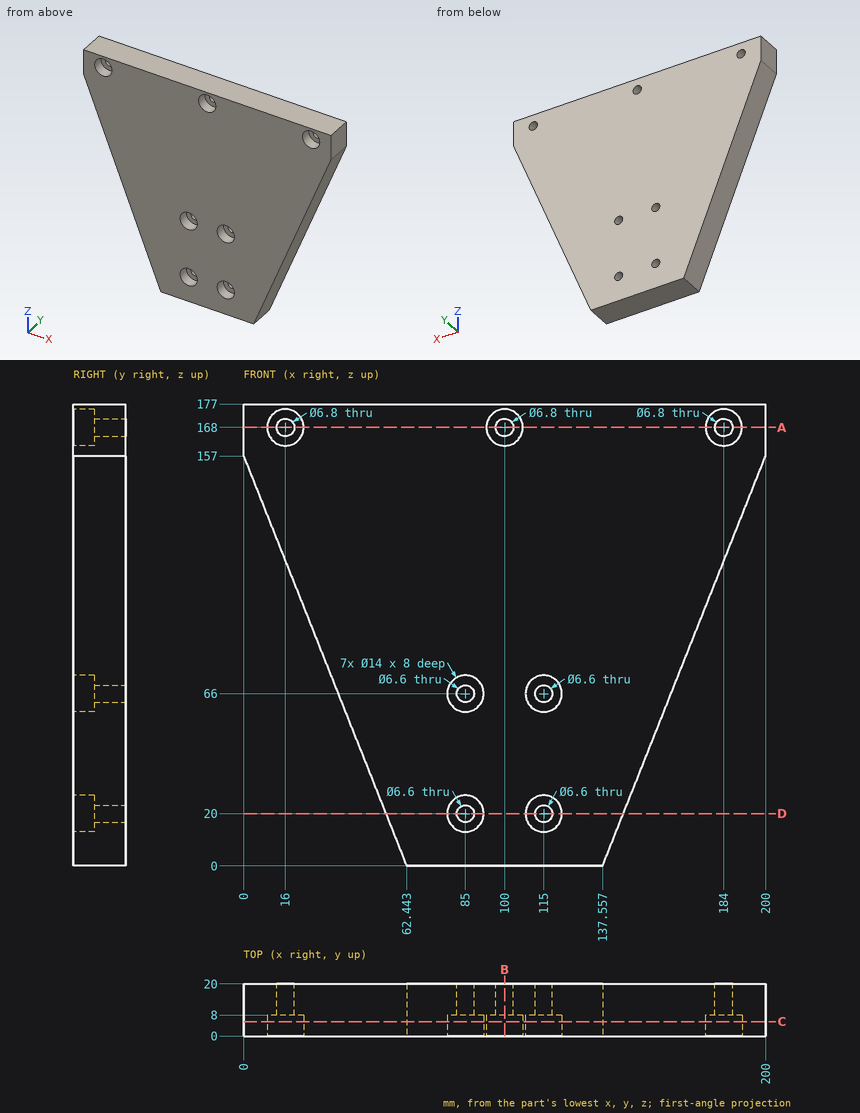
The drawing under review shows one solid part. Ordinate dimensions are in mm from its lowest x, y, z. Round coordinates to 2 decimals unless told otherwise and drop trailing zeros. Loops run counter-clockwise (first coordinate to the right, second up) from the corner with the lowest first, then second, coordinate; pieces in that order, holes last. Notation, with made-up numbers: (-7, 10.5) - (24, 10.5) arc R28 cw to (24, 32.5) - close; hole circle Ø10 at (24, 1). An arc over 180 degrees is marked (long way). Use a Markdown table: item, result. Add a question column.
Q1. Add section B-B (x = 100). State the section outline as (y, z) points, plus the area to 3 significant figures.
Q2. Add section A-A (z = 168). State the section outline as (x, y) points, plus the area to 3 significant figures.
Q3. Add section C-C (y = 5.5). State the section outline as (x, z) points, plus the area to 3 significant figures.
Q4. Insertion check: pin 1 Ø9 at (x, z) = (184, 168) entering from -Y; pin 2 Ø2 at (y, z) = (5, 107.5) entering from -X; pin 3 Ø1.5 at (y, z) = (7.5, 57.5) entering from +X (1 decimal); pin 4 Ø5.5 at (x, z) = (85, 66) entering from +Y. Each pin has a flat end and moves straight along its axis. Give the tip position at first contact, or say it passes through.
Q5. For probe 1 along X at (y, z) = (16.25, 168); probe 2 along X at (y, z) = (5.5, 24.5); probe 3 along Z at (x, y) = (97, 2) (1 decimal), list the stretches that pass through material, from the lowest coordinate up.
Q6. Add section D-D (z = 20). State the section outline as (x, y) points.
Worked answers:
| question | item | result |
|---|---|---|
| 1 | outline | (0, 0) - (20, 0) - (20, 164.6) - (8, 164.6) - (8, 161) - (0, 161) - close; (0, 175) - (8, 175) - (8, 171.4) - (20, 171.4) - (20, 177) - (0, 177) - close |
| 1 | area | 3,350 mm² |
| 2 | outline | (0, 0) - (9, 0) - (9, 8) - (12.6, 8) - (12.6, 20) - (0, 20) - close; (19.4, 8) - (23, 8) - (23, 0) - (93, 0) - (93, 8) - (96.6, 8) - (96.6, 20) - (19.4, 20) - close; (103.4, 8) - (107, 8) - (107, 0) - (177, 0) - (177, 8) - (180.6, 8) - (180.6, 20) - (103.4, 20) - close; (187.4, 8) - (191, 8) - (191, 0) - (200, 0) - (200, 20) - (187.4, 20) - close |
| 2 | area | 3,420 mm² |
| 3 | outline | (0, 157) - (62.44, 0) - (137.56, 0) - (200, 157) - (200, 177) - (0, 177) - close; hole circle Ø14 at (16, 168); hole circle Ø14 at (85, 20); hole circle Ø14 at (85, 66); hole circle Ø14 at (100, 168); hole circle Ø14 at (115, 20); hole circle Ø14 at (115, 66); hole circle Ø14 at (184, 168) |
| 3 | area | 24,500 mm² |
| 4 | pin 1 | y = 8 |
| 4 | pin 2 | x = 19.29 |
| 4 | pin 3 | x = 160.7 |
| 4 | pin 4 | through |
| 5 | probe 1 | 0 to 12.6, 19.4 to 96.6, 103.4 to 180.6, 187.4 to 200 |
| 5 | probe 2 | 52.7 to 79.64, 90.36 to 109.64, 120.36 to 147.3 |
| 5 | probe 3 | 0 to 161.7, 174.3 to 177 |
| 6 | outline | (54.49, 0) - (78, 0) - (78, 8) - (81.7, 8) - (81.7, 20) - (54.49, 20) - close; (88.3, 8) - (92, 8) - (92, 0) - (108, 0) - (108, 8) - (111.7, 8) - (111.7, 20) - (88.3, 20) - close; (118.3, 8) - (122, 8) - (122, 0) - (145.51, 0) - (145.51, 20) - (118.3, 20) - close |
